from build123d import *

# Parameters (mm, degrees)
ESQUISSE4_R      = 1.5
EXTRUSION3_DEPTH = 19
ESQUISSE3_R      = 2
EXTRUSION4_DEPTH = 7


with BuildPart() as part:
    # Esquisse1 → Révolution1 (revolve)
    with BuildSketch(Plane.XY):
        Polygon((19, -12), (27, -12), (27, -8), (17, -8), (17, -6), (15, -6), (15, -20), (9, -20), (9, -24), (19, -24), align=None)
    revolve(axis=Axis((0, 0, 0), (0, -1, 0)))

    # Esquisse4 → Extrusion3 (cut, through all)
    with BuildSketch(Plane.XZ.offset(24)):
        with Locations((0, 13)):
            Circle(ESQUISSE4_R)
        with Locations((13, 0)):
            Circle(ESQUISSE4_R)
        with Locations((0, -13)):
            Circle(ESQUISSE4_R)
        with Locations((-13, 0)):
            Circle(ESQUISSE4_R)
    extrude(amount=-EXTRUSION3_DEPTH, mode=Mode.SUBTRACT)

    # Esquisse3 → Extrusion4 (cut, through all)
    with BuildSketch(Plane.XZ.offset(12)):
        with Locations((24, 0)):
            Circle(ESQUISSE3_R)
        with Locations((0, 24)):
            Circle(ESQUISSE3_R)
        with Locations((0, -24)):
            Circle(ESQUISSE3_R)
        with Locations((-24, 0)):
            Circle(ESQUISSE3_R)
    extrude(amount=-EXTRUSION4_DEPTH, mode=Mode.SUBTRACT)


solid = part.part
Geometry: final body of the model. Coordinates: model frame, mm. A direction names the side the tool comes from. Coordinates: 2 decimals unless noted, no trailing zeros. Order: outer loops, then holes, each group sorted by start corner. A loop starts at its lowest first (then second) coordinate and runs counter-clockwise, first axis right, second up. Notation, with made-up numbers: (25.25, 61.5) - (81.25, 61.5) arc R14 ccw to (81.25, 82.5) - close; hole circle Ø4 at (54, 36). An arc over 180 degrees is marked (long way). Use one line per item in the form item = value.
1) Set-up query: faces 5 (the face through (18, -12, -8)), 6 (the face through (-0.325, -22.028, 11.536)), 7 (the face through (18, -8, 0)). Return all of +Z, -Z, +X, -X, +Y, -Y with unobstructed straight access to the full face (end or side cutting, diameter ignored); none if empty.
Solutions:
face_5 = -Y
face_6 = +Y, -Y
face_7 = +Y
2) Section A-A (z = 13). Return loops of the section in (x, y), then the cut area to 3 significant figures.
Solutions:
outline = (-23.66, -12) - (-13.86, -12) - (-13.86, -24) - (-1.5, -24) - (-1.5, -20) - (-7.48, -20) - (-7.48, -6) - (-10.95, -6) - (-10.95, -8) - (-23.66, -8) - close; (1.5, -24) - (13.86, -24) - (13.86, -12) - (23.66, -12) - (23.66, -8) - (10.95, -8) - (10.95, -6) - (7.48, -6) - (7.48, -20) - (1.5, -20) - close
area = 344 mm^2
3) Pin query (flat end, axial travel): pin 1 (3.5 mm diameter, centred on x = -24, z = 0, fed in from -Y); pin 2 (24 mm diameter, centred on x = 0, z = 0, fed in from +Y); pin 3 (6.5 mm diameter, centred on x = 0, z = 24, fed in from -Y); pin 4 (2 mm diameter, centred on y = -9.5, z = 17, fed in from +X). Return the tip coordinate at first contact, or that it passes through.
Solutions:
pin_1 = through
pin_2 = -20
pin_3 = -12
pin_4 = 21.75
4) Section B-B (y = -15.75). Return loops of the section in (x, z), then the cut area to 3 significant figures.
Solutions:
outline = circle Ø38 at (0, 0); hole circle Ø30 at (0, 0)
area = 427 mm^2
5) Mould query, pull axis X, two halves, no side actions, for faces 1 (the face through (8.767, -17.916, -16.856)), 2 (the face through (6, -6, -14)), 3 (the face through (0.923, -10.028, 22.226)), 4 (the face through (-26, -10, 0)). Classes: +X half, -X half, draft (parallel to the pull), parting line (faces both ways), or undercut.
Solutions:
face_1 = parting line
face_2 = draft
face_3 = undercut
face_4 = undercut
6) Ray query, L1, parallel to Z at x = 0, y = -21.5; L2, parallel to Z at x = 0, y = -10; L3, parallel to Y at x = 10, z = -22. Return the intervals inside material, ascending.
Solutions:
L1 = -19 to -14.5, -11.5 to -9, 9 to 11.5, 14.5 to 19
L2 = -27 to -26, -22 to -15, 15 to 22, 26 to 27
L3 = -12 to -8
7) Section C-C (x = 0). State how many separate pieces and enclosed holes the cut face has, then the cut area to 3 significant figures.
Solutions:
separate_pieces = 6
enclosed_holes = 0
area = 192 mm^2
